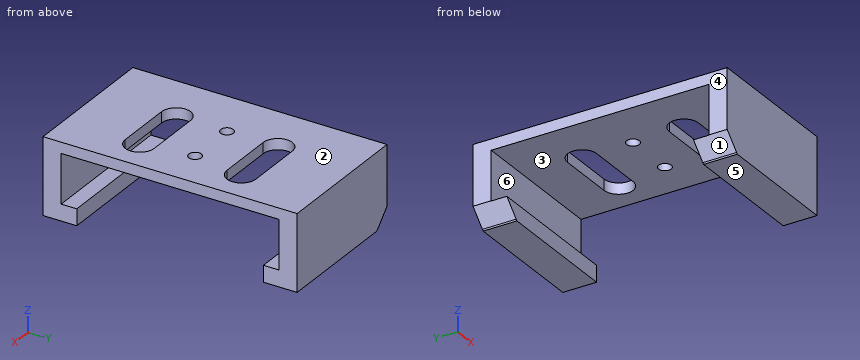
Autodesk Fusion 360 part; units mm, degrees
sketch "Sketch1" plane through (0, 0, 0) normal (0, 0, 1) x (1, 0, 0)
  line L0 (30, 25.7) -> (-30, 25.7)
  line L1 (-30, 25.7) -> (-30, -25.7)
  line L2 (-30, -25.7) -> (30, -25.7)
  line L3 (30, -25.7) -> (30, 25.7)
  line L4 (30, -30) -> (-30, -30)
  line L5 (-30, -35) -> (-30, 35)
  line L6 (-30, 30) -> (30, 30)
  line L7 (30, 30) -> (30, -30)
  line L8 (-30, 35) -> (27, 35)
  line L9 (35, 27) -> (35, -27)
  line L10 (-30, -35) -> (27, -35)
  arc A0 (35, 27) -> (27, 35) centre (27, 27) ccw
  arc A1 (27, -35) -> (35, -27) centre (27, -27) ccw
  circle A2 centre (-20, 0) radius 1.75
  line L11 (-19.9675, 10) -> (-4, 10)
  arc A3 (-4, 10) -> (-4, 18) centre (-4, 14) ccw
  line L12 (-4, 18) -> (-19.9675, 18)
  arc A4 (-19.9675, 18) -> (-19.9675, 10) centre (-19.9675, 14) ccw
  line L13 (-19.9675, 14) -> (-4, 14) construction
  line L14 (1.75, 0) -> (22.5, 0)
  line L15 (-19.9675, -10) -> (-4, -10)
  arc A5 (-19.9675, -10) -> (-19.9675, -18) centre (-19.9675, -14) ccw
  line L16 (-4, -18) -> (-19.9675, -18)
  arc A6 (-4, -18) -> (-4, -10) centre (-4, -14) ccw
  circle A7 centre (-6, 0) radius 1.75
  dimension "d1" = 60
  dimension "d2" = 51.4
  dimension "d3" = 60
  dimension "d6" = 8
  dimension "d15" = 3.5
  dimension "d37" = 3.5
extrude "Extrude1" add sketch "Sketch1" along normal blind 4.5 contours L3 L4 L5 L6 L7 L8 L9 L10 A0 A1 | L0 L5 L6 L7 | L2 L4 L5 L7
extrude "Extrude2" add sketch "Sketch1" along normal blind 18 contours L3 L4 L5 L6 L7 L8 L9 L10 A0 A1
extrude "Extrude3" add sketch "Sketch1" along normal blind 21 and the other way blind -18
sketch "Sketch2" plane through (0, -35, 0) normal (0, -1, 0) x (1, 0, 0)
  line L0 (-30, 0) -> (27, 0)
  line L1 (27, 0) -> (27, 21)
  line L2 (27, 21) -> (-30, 21)
  line L3 (-30, 21) -> (-30, 0)
  line L4 (-30, 0) -> (-34.45, 0)
  line L5 (-34.45, 0) -> (-34.45, 4.55)
  line L6 (-30, 0) -> (-30.316, 0.3196)
  line L7 (-30.316, 0.3196) -> (-34.45, 4.55)
  line L8 (-34.45, 4.55) -> (-34.45, 21)
  line L9 (-34.45, 21) -> (-30, 21)
  line L10 (-30, 0) -> (-30, 5.5)
  line L11 (-30, 5.5) -> (-34.45, 5.5)
  line L12 (-34.45, 4.55) -> (-29.5, 4.55)
  dimension "d17" = 4.45
  dimension "d18" = 4.55
  dimension "d25" = 5.5
extrude "Extrude4" add sketch "Sketch2" against normal blind 5 contours L3 L6 L7 L10 L12 | L3 L8 L10 L11 L12 | L3 L8 L9 L11
extrude "Extrude5" add sketch "Sketch2" along normal blind -70 and the other way blind 65 contours L3 L6 L7 L10 L12 | L3 L8 L10 L11 L12 | L3 L8 L9 L11
extrude "Extrude6" add sketch "Sketch2" against normal blind 9.3 contours L3 L6 L7 L10 L12
extrude "Extrude7" add sketch "Sketch2" along normal blind -65 and the other way blind 60.7 contours L3 L6 L7 L10 L12
extrude "Extrude8" add 1 faces at (-30, -10, 19) along direction (-1, 0, 0) blind 4.45
extrude "Extrude9" cut 2 faces at (-32.9667, -28.5667, 4.55) (-32.9667, 27.1333, 4.55) along direction (0, 0, -1) blind 0.05
sketch "Sketch3" plane through (0, 0, 21) normal (0, 0, 1) x (-1, 0, 0)
  circle A0 centre (20, 0) radius 1.75
  arc A1 (19.9675, -18) -> (19.9675, -10) centre (19.9675, -14) ccw
  line L0 (19.9675, -18) -> (4, -18)
  arc A2 (4, -10) -> (4, -18) centre (4, -14) ccw
  line L1 (4, -10) -> (19.9675, -10)
  arc A3 (19.9675, 10) -> (19.9675, 18) centre (19.9675, 14) ccw
  line L2 (19.9675, 10) -> (4, 10)
  arc A4 (4, 18) -> (4, 10) centre (4, 14) ccw
  line L3 (4, 18) -> (19.9675, 18)
  line L4 (34.45, 35) -> (-27, 35)
  arc A5 (-27, 35) -> (-35, 27) centre (-27, 27) ccw
  line L5 (-35, 27) -> (-35, -27)
  arc A6 (-35, -27) -> (-27, -35) centre (-27, -27) ccw
  line L6 (-27, -35) -> (34.45, -35)
  line L7 (34.45, -35) -> (34.45, 35)
  line L8 (-5, -40) -> (-40, -40)
  line L9 (-40, -40) -> (-40, 40)
  line L10 (-40, 40) -> (-5, 40)
  line L11 (-5, 40) -> (-5, -40)
  circle A7 centre (6, 0) radius 1.75
extrude "Extrude10" cut sketch "Sketch3" against normal blind 40 contours L4 A5 L5 A6 L6 L11 | L4 A5 L5 A6 L6 L8 L9 L10 L11
The listing builds one solid part. Answer for the finished solid, in the listing's coordinates (mm). Face numbers are marked on the shaded views. A direction names the side the tool comes from. Coordinates: 2 decimals unless noted, no trailing zeros. Loops run counter-clockwise (first coordinate to the right, second up) from the corner with the lowest first, then second, coordinate; pieces in that order, holes last. Notation, with made-up numbers: M 10,79 L 68,79 A13 ccw 68,89 Z; hole C 89.25,52 d4. An arc over 180 degrees is marked long. Answer as CSV lines item,"result". Start each with the question number.
(1) The part is cut by section C-C (z = 6.75). Give the vertices of the cut face in (x, y), and give its area (4 significant figures).
(2) The part is cut by section A-A (y = 14). Give the vertices of the cut face in (x, z), and give its area (3 significant figures).
(3) The part is cut by section D-D (y = 0). Give the vertices of the cut face in (x, z).
(4) Given pin 1 (12 mm diameter, centred on x = -11, y = 10, fed in from -Z); pin 2 (2 mm diameter, centred on x = -6, y = 0, fed in from +Z), each flat-ended and moving along its own axis, determine where each tip first touches the part or whether it passes through.
(5) The mould has two halves that part along Z. Classify the marked faces 1, 2, 3 and 4: pulls with the +Z half, pulls with the -Z half, needs draft (parallel to the pull), parting line crosses it, or undercut.
(6) Find the intervals of material crossed by L1, parallel to Y at x = -26, z = 11.75; L2, parallel to Y at x = -15, z = 3.25; L3, parallel to Y at x = -20, z = 19.2, in increasing order. Write a range as [from, to].
(7) For the marked faces 5 and 6, determine the directions among +Z, -Z, +X, -X, +Y, -Y from which every point of the face is accessible in a straight line to the end or side of a thin tool.
(8) The part is cut by section B-B (x = -14.5). Give the vertices of the cut face in (y, z), and give its area (3 significant figures).
Determined:
1,outline,"M -34.45,-35 L 5,-35 L 5,-30 L -34.45,-30 Z; M -34.45,30 L 5,30 L 5,35 L -34.45,35 Z"
1,area,"394.5 mm2"
2,outline,"M -34.45,18 L -23.97,18 L -23.97,21 L -34.45,21 Z; M 0,18 L 5,18 L 5,21 L 0,21 Z"
2,area,"46.4 mm2"
3,outline,"M -34.45,18 L -21.75,18 L -21.75,21 L -34.45,21 Z; M -18.25,18 L -7.75,18 L -7.75,21 L -18.25,21 Z; M -4.25,18 L 5,18 L 5,21 L -4.25,21 Z"
4,pin 1,"z = 18"
4,pin 2,"through"
5,face 1,"pulls with the -Z half"
5,face 2,"pulls with the +Z half"
5,face 3,"undercut"
5,face 4,"needs draft"
6,L1,"[-35, -30], [30, 35]"
6,L2,"[-35, -25.7], [25.7, 35]"
6,L3,"[-35, -18], [-10, -1.75], [1.75, 10], [18, 35]"
7,face 5,"-Z, +X, -X, +Y, -Y"
7,face 6,"+X, -X"
8,outline,"M -35,0 L -25.7,0 L -25.7,4.5 L -30,4.5 L -30,18 L -18,18 L -18,21 L -35,21 Z; M -10,18 L 10,18 L 10,21 L -10,21 Z; M 18,18 L 30,18 L 30,4.5 L 25.7,4.5 L 25.7,0 L 35,0 L 35,21 L 18,21 Z"
8,area,"381 mm2"
